Study the drawing (mm; zero at the part's minimum x, y, z) and answer. A direction names the side the tool comes from. Give positions to 0.01 mm unless a question says otherwise; leave off trailing zeros. Write each loop counter-clockwise with the first axis right and the second up, starting at its lowest first coordinate (ties: lowest second). Pieces come first, ordered by that corner, then holes. Notation, with made-up numbers: (55, -38) - (79, -38) arc R14 ccw to (79, -30) - close; hole circle Ø7 at (10.5, 29). An arc over 180 degrees is marked (long way). Return JSON: item names as keys, results as strings.
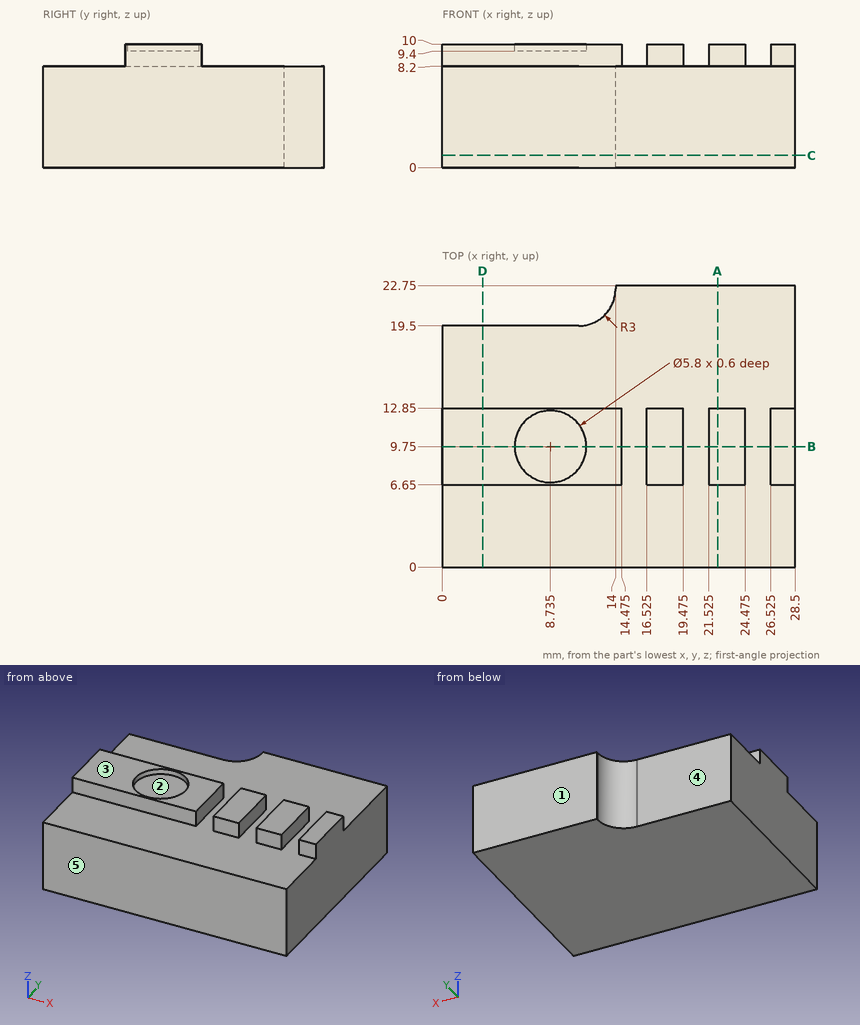
Item 1: The mould has two halves that part along Y. Classify the marked faces 1, 2 and 3: +Y half, -Y half, draft (parallel to the pull), parting line (faces both ways), or undercut.
Answer below:
{"face 1": "+Y half", "face 2": "undercut", "face 3": "draft"}
Item 2: Consider L1, parallel to X at y = 11.5, z = 9.25 (3 decimals); L2, parallel to Y at x = 7.75, z = 7; L3, parallel to Z at x = 25, y = 7. Determine where each line is inside the solid, lowest interval first.
Answer below:
{"L1": "x = 0 to 14.475, 16.525 to 19.475, 21.525 to 24.475, 26.525 to 28.5", "L2": "y = 0 to 19.5", "L3": "z = 0 to 8.2"}
Item 3: A cutting plane is placed at A-A on x = 22.25. Determine the outline of the cut face in (y, z), then the cut area to 3 significant figures.
Answer below:
{"outline": "(0, 0) - (22.75, 0) - (22.75, 8.2) - (12.85, 8.2) - (12.85, 10) - (6.65, 10) - (6.65, 8.2) - (0, 8.2) - close", "area": "198 mm²"}
Item 4: A cutting plane is placed at B-B on y = 9.75. Determine the outline of the cut face in (x, z) (3 decimals).
Answer below:
{"outline": "(0, 0) - (28.5, 0) - (28.5, 10) - (26.525, 10) - (26.525, 8.2) - (24.475, 8.2) - (24.475, 10) - (21.525, 10) - (21.525, 8.2) - (19.475, 8.2) - (19.475, 10) - (16.525, 10) - (16.525, 8.2) - (14.475, 8.2) - (14.475, 10) - (11.635, 10) - (11.635, 9.4) - (5.835, 9.4) - (5.835, 10) - (0, 10) - close"}
Item 5: A cutting plane is placed at D-D on x = 3.25. Determine the outline of the cut face in (y, z), then the cut area to 3 significant figures.
Answer below:
{"outline": "(0, 0) - (19.5, 0) - (19.5, 8.2) - (12.85, 8.2) - (12.85, 10) - (6.65, 10) - (6.65, 8.2) - (0, 8.2) - close", "area": "171 mm²"}
Item 6: Flat-ended cylindrical pins translate along their axes: P1, Ø5, axis at x = 3.5, y = 15, coming from the +Z side; P2, Ø1.4, axis at x = 9.5, z = 9, coming from the -Y side; P3, Ø4, axis at x = 3, z = 3, coming from the +Y side; P4, Ø3, axis at x = 9.5, y = 10.5, coming from the +Z side. Find the tip coordinate at first contact, or state that the pin passes through.
Answer below:
{"P1": "stops at z = 10", "P2": "stops at y = 6.65", "P3": "stops at y = 19.5", "P4": "stops at z = 9.4"}
Item 7: A cutting plane is placed at C-C on z = 1. Determine the outline of the cut face in (x, y).
Answer below:
{"outline": "(0, 0) - (28.5, 0) - (28.5, 22.75) - (14, 22.75) - (14, 22.5) arc R3 cw to (11, 19.5) - (0, 19.5) - close"}
Item 8: For the marked faces 4 and 5, determine the directions among +Z, -Z, +X, -X, +Y, -Y from which every point of the face is accessible in a straight line to the end or side of a thin tool.
Answer below:
{"face 4": "+Z, -Z, -X, +Y", "face 5": "+Z, -Z, +X, -X, -Y"}
